Here's how the part is built. I have some questions about the finished solid (model axes, mm). Face numbers are marked on the shaded views. A direction names the side the tool comes from. Round coordinates to 2 decimals unless told otherwise and drop trailing zeros. Write each loop counter-clockwise with the first axis right and the second up, starting at its lowest first coordinate (ties: lowest second). Pieces come first, ordered by that corner, then holes. Notation, with made-up numbers: (-6.75, 65) -> (17.25, 65) arc R22 cw to (17.25, 81) -> close; hole circle Ø11 at (-29, -31.75). An arc over 180 degrees is marked (long way). Answer in a Markdown table with one row per item.
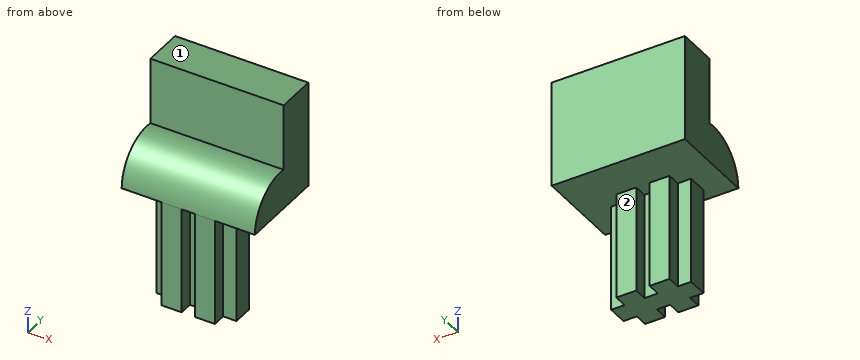
from build123d import *

# Parameters (mm, degrees)
F1_DEPTH = 10
F2_W     = 2
F2_H     = 8
F3_DEPTH = 6.501
F4_W     = 1
F4_H     = 1
F5_DEPTH = 8


with BuildPart() as f1:
    # F0 (on Right) → F1 (new body)
    with BuildSketch(Plane.YZ):
        with BuildLine():
            Line((-3.5, -8), (0, -8))
            Line((0, -8), (0, 0))
            Line((0, 0), (3, 0))
            Line((3, 0), (3, 8))
            Line((3, 8), (0, 8))
            Line((0, 8), (0, 3))
            ThreePointArc((0, 3), (-2.439902, 2.304886), (-3.5, 0))
            Line((-3.5, 0), (-3.5, -8))
        make_face()
    extrude(amount=F1_DEPTH)

    # F2 (on face) → F3 (cut, through all)
    with BuildSketch(Plane.XZ.offset(3.5)):
        with Locations((1, -4)):
            Rectangle(F2_W, F2_H)
        with Locations((9, -4)):
            Rectangle(F2_W, F2_H)
    extrude(amount=-F3_DEPTH, mode=Mode.SUBTRACT)

    # F4 (on face) → F5 (cut)
    with BuildSketch(Plane(origin=(0, 0, -8), x_dir=(1, 0, 0), z_dir=(0, 0, -1))):
        with Locations((2.5, 3)):
            Rectangle(F4_W, F4_H)
        with Locations((2.5, 0.5)):
            Rectangle(F4_W, F4_H)
        with Locations((7.5, 0.5)):
            Rectangle(F4_W, F4_H)
        with Locations((7.5, 3)):
            Rectangle(F4_W, F4_H)
        with Locations((5, 3)):
            Rectangle(F4_W, F4_H)
        with Locations((5, 0.5)):
            Rectangle(F4_W, F4_H)
    extrude(amount=-F5_DEPTH, mode=Mode.SUBTRACT)


solid = f1.part
1) I need wall thicknesses on line 1 (X direction, y = -2.75, z = -6.25); line 2 (Y direction, x = 6, z = 4.5); line 3 (Y direction, x = 4.25, z = -5.75). Which ranges of each line are inside material? Lowest first, please. Write a range as [from, to].
Response:
| item | result |
|---|---|
| line 1 | x = [3, 4.5], [5.5, 7] |
| line 2 | y = [0, 3] |
| line 3 | y = [-3.5, 0] |
2) Which directions (+Z, -Z, +X, -X, +Y, -Y) give clear straight access to the entire face, cutting with the end or side of a thin tool? Please do the marked faces 1 and 2.
Response:
| item | result |
|---|---|
| face 1 | +Z, +X, -X, +Y, -Y |
| face 2 | -Z, +X, -X, +Y |
3) I want a section at A-A, the plane x = 2.25. List the corners of the cut face in (y, z) for me, and give its area (3 significant figures).
Response:
| item | result |
|---|---|
| outline | (-3.5, 0) -> (-2.5, 0) -> (-2.5, -8) -> (-1, -8) -> (-1, 0) -> (3, 0) -> (3, 8) -> (0, 8) -> (0, 3) arc R3.04 ccw to start |
| area | 44.6 mm^2 |
4) I want a section at D-D, the plane x = 6. List the corners of the cut face in (y, z) for me.
Response:
| item | result |
|---|---|
| outline | (-3.5, -8) -> (0, -8) -> (0, 0) -> (3, 0) -> (3, 8) -> (0, 8) -> (0, 3) arc R3.04 ccw to (-3.5, 0) -> close |
5) I want a section at B-B, the plane z = -1.5. List the corners of the cut face in (x, y) for me, and give its area (3 significant figures).
Response:
| item | result |
|---|---|
| outline | (2, -2.5) -> (3, -2.5) -> (3, -3.5) -> (4.5, -3.5) -> (4.5, -2.5) -> (5.5, -2.5) -> (5.5, -3.5) -> (7, -3.5) -> (7, -2.5) -> (8, -2.5) -> (8, -1) -> (7, -1) -> (7, 0) -> (5.5, 0) -> (5.5, -1) -> (4.5, -1) -> (4.5, 0) -> (3, 0) -> (3, -1) -> (2, -1) -> close |
| area | 15.0 mm^2 |
6) For pin 1 (2 mm diameter, centred on x = 8.5, z = -3, fed in from -Y); pin 2 (0.8 mm diameter, centred on y = -0.5, z = -5, fed in from -X); pin 3 (1.6 mm diameter, centred on x = 4, z = -4, fed in from +Y); pin 4 (2 mm diameter, centred on x = 7, z = -0.5, fed in from +Y), each with a flat end and sliding along its axis, tell me the tip position at first contact or that it passes through.
Response:
| item | result |
|---|---|
| pin 1 | stops at y = -2.5 |
| pin 2 | stops at x = 3 |
| pin 3 | stops at y = 0 |
| pin 4 | stops at y = 3 |
7) I want a section at C-C, the plane y = -0.25. List the corners of the cut face in (x, z) for me, and give its area (3 significant figures).
Response:
| item | result |
|---|---|
| outline | (0, 0) -> (3, 0) -> (3, -8) -> (4.5, -8) -> (4.5, 0) -> (5.5, 0) -> (5.5, -8) -> (7, -8) -> (7, 0) -> (10, 0) -> (10, 3.03) -> (0, 3.03) -> close |
| area | 54.3 mm^2 |
